For this review, take the finished solid that the model builds, in its own axes (mm). Coordinates: 2 decimals unless noted, no trailing zeros. Loops run counter-clockwise (first coordinate to the right, second up) from the corner with the lowest first, then second, coordinate; pieces in that order, holes last.
1. Clearance check with a flat-ended pin moving along its axis: P1, Ø2, axis at x = 115, z = -52, coming from the -Y side. State where the tip first meets the part, or that it passes through.
2. To check wall thickness, follow probe 1 along X at (y, z) = (2.1, 50.5); probe 2 along X at (y, z) = (2, -58.5); probe 3 along Z at (x, y) = (85.5, 0.9). State the ranges of each line that lie inside material, in increasing order.
3. Take a section at B-B, the plane x = -52.5. State the section outline as (y, z) points.
4. Take a section at A-A, the plane z = 71. State the section outline as (x, y) points.
```python
from build123d import *

# Parameters (mm, degrees)
F0_R            = 175
F1_DEPTH        = 3
F3_DEPTH        = 3.001
F3_COPIES_COUNT = 30


# Not quite as in the source:
# - a pattern or mirror of a feature is missing from the dataset's text; its kind, count and spacing are read off the source's solid


with BuildPart() as f1:
    # F0 (on Front) → F1 (new body)
    with BuildSketch(Plane.XZ):
        Circle(F0_R)
    extrude(amount=-F1_DEPTH)

    # F2 (on face) → F3 (cut, through all)
    with BuildSketch(Plane.XZ):
        with BuildLine():
            ThreePointArc((-5.1165300167, 174.9251872104), (-7.1549450675, 174.8536724266), (-9.1923881554, 174.758404662))
            Line((-9.1923881554, 174.758404662), (4.9497474683, 160.6162690382))
            Line((4.9497474683, 160.6162690382), (7.0710678119, 162.7375893818))
            Line((7.0710678119, 162.7375893818), (-5.1165300167, 174.9251872104))
        make_face()
    f3 = extrude(amount=-F3_DEPTH, mode=Mode.SUBTRACT)

    # F3_copies: F3 ×30 about axis
    f3_copies_axis = Axis((0, 0, 0), (0, 1, 0))
    for i in range(1, F3_COPIES_COUNT):
        add(f3.rotate(f3_copies_axis, i * 360 / F3_COPIES_COUNT), mode=Mode.SUBTRACT)


solid = f1.part
```
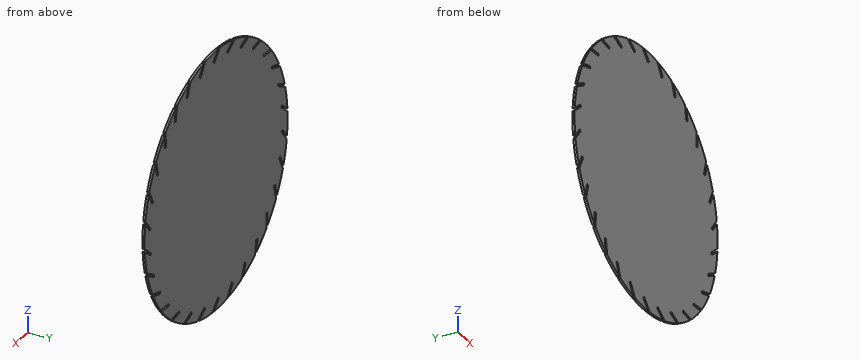
Results list:
1. P1: stops at y = 0
2. probe 1: x = -167.56 to -165.37, -158.76 to 157.12, 160.49 to 167.56
2. probe 2: x = -164.93 to -164.57, -161.2 to 164.93
2. probe 3: z = -152.69 to 152.69
3. outline: (0, -166.94) - (3, -166.94) - (3, 166.94) - (0, 166.94) - close
4. outline: (-159.95, 0) - (159.95, 0) - (159.95, 3) - (-159.95, 3) - close
